Model file for the job. Use its own axes, mm. Face numbers are marked on the shaded views. A direction names the side the tool comes from. Round coordinates to 2 decimals unless told otherwise and drop trailing zeros. Order: outer loops, then holes, each group sorted by start corner. A loop starts at its lowest first (then second) coordinate and runs counter-clockwise, first axis right, second up. Notation, with made-up numbers: (-15, -15.5) - (26, -15.5) arc R20 cw to (26, 13.5) - close; hole circle Ø10 at (19, -28.5). An arc over 180 degrees is marked (long way). Write item = value, one per line.
```python
from build123d import *

# Parameters (mm, degrees)
SKETCH2_R                      = 70
BOSS_EXTRUDE1_DEPTH            = 15
CBORE_FOR_M5_SHCS1_D           = 5.5
CBORE_FOR_M5_SHCS1_CBORE_D     = 10
CBORE_FOR_M5_SHCS1_CBORE_DEPTH = 5
SKETCH23_R                     = 20.1
SKETCH23_R_2                   = 18.5
BOSS_EXTRUDE2_DEPTH            = 19
SKETCH24_R                     = 18.5
CUT_EXTRUDE4_DEPTH             = 101.801785698
SKETCH25_R                     = 22.2
SKETCH25_R_2                   = 20.1
BOSS_EXTRUDE3_DEPTH            = 4
FILLET2_R                      = 2


with BuildPart() as part:
    # Sketch2 → Boss-Extrude1 (new body)
    with BuildSketch(Plane(origin=(0, 0, 0), x_dir=(1, 0, 0), z_dir=(0, 1, 0))):
        with Locations(Location((0, 0, 0), (0, 0, 270))):
            Circle(SKETCH2_R)
    extrude(amount=BOSS_EXTRUDE1_DEPTH)

    # CBORE for M5 SHCS1 (through all)
    with Locations(Plane(origin=(0, 15, 0), x_dir=(1, 0, 0), z_dir=(0, 1, 0))):
        with Locations((0, 60), (60, 0), (-60, 0), (0, -60)):
            CounterBoreHole(CBORE_FOR_M5_SHCS1_D / 2, CBORE_FOR_M5_SHCS1_CBORE_D / 2, CBORE_FOR_M5_SHCS1_CBORE_DEPTH)

    # Sketch23 → Boss-Extrude2 (add)
    with BuildSketch(Plane(origin=(0, 15, 0), x_dir=(1, 0, 0), z_dir=(0, 1, 0))):
        with Locations(Location((0, 0, 0), (0, 0, 270))):
            Circle(SKETCH23_R)
        with Locations(Location((0, 0, 0), (0, 0, 270))):
            Circle(SKETCH23_R_2, mode=Mode.SUBTRACT)
    extrude(amount=BOSS_EXTRUDE2_DEPTH)

    # Sketch24 → Cut-Extrude4 (cut, through all)
    with BuildSketch(Plane(origin=(0, 15, 0), x_dir=(1, 0, 0), z_dir=(0, 1, 0))):
        with Locations(Location((0, 0, 0), (0, 0, 270))):
            Circle(SKETCH24_R)
    extrude(amount=-CUT_EXTRUDE4_DEPTH, mode=Mode.SUBTRACT)

    # Sketch25 → Boss-Extrude3 (add)
    with BuildSketch(Plane(origin=(0, 15, 0), x_dir=(1, 0, 0), z_dir=(0, 1, 0))):
        with Locations(Location((0, 0, 0), (0, 0, 270))):
            Circle(SKETCH25_R)
        with Locations(Location((0, 0, 0), (0, 0, 270))):
            Circle(SKETCH25_R_2, mode=Mode.SUBTRACT)
    extrude(amount=BOSS_EXTRUDE3_DEPTH)

    # Fillet2
    # the kernel refuses this fillet: 2 mm, written as the material it adds along each edge
    with BuildSketch(Plane(origin=(0, 15, 0), x_dir=(0, 0, 1), z_dir=(-1, 0, 0))) as fillet2_piece_1:
        with BuildLine():
            CenterArc((22.2 + FILLET2_R, FILLET2_R), FILLET2_R, 180, 90)
            Line((22.2, FILLET2_R), (22.2, 0))
            Line((22.2, 0), (22.2 + FILLET2_R, 0))
        make_face()
    revolve(axis=Axis((0, 15, 0), (0, 1, 0)))
    # the kernel refuses this fillet: 2 mm, written as the material it takes off along each edge
    with BuildSketch(Plane(origin=(0, 0, 0), x_dir=(0, 0, 1), z_dir=(-1, 0, 0))) as fillet2_2_piece_1:
        with BuildLine():
            CenterArc((70 - FILLET2_R, FILLET2_R), FILLET2_R, 270, 90)
            Line((70 - FILLET2_R, 0), (70, 0))
            Line((70, 0), (70, FILLET2_R))
        make_face()
    revolve(axis=Axis((0, 0, 0), (0, 1, 0)), mode=Mode.SUBTRACT)
    with BuildSketch(Plane(origin=(0, 34, 0), x_dir=(0, 0, 1), z_dir=(-1, 0, 0))) as fillet2_2_piece_2:
        with BuildLine():
            CenterArc((18.1, -1.959591794), FILLET2_R, 0, 78.463040967)
            Line((20.1, -1.959591794), (20.1, 0))
            Line((20.1, 0), (18.5, 0))
        make_face()
    revolve(axis=Axis((0, 34, 0), (0, 1, 0)), mode=Mode.SUBTRACT)
    with BuildSketch(Plane(origin=(0, 15, 0), x_dir=(0, 0, 1), z_dir=(-1, 0, 0))) as fillet2_2_piece_3:
        with BuildLine():
            CenterArc((70 - FILLET2_R, -FILLET2_R), FILLET2_R, 0, 90)
            Line((70 - FILLET2_R, 0), (70, 0))
            Line((70, 0), (70, -FILLET2_R))
        make_face()
    revolve(axis=Axis((0, 15, 0), (0, 1, 0)), mode=Mode.SUBTRACT)


solid = part.part
```
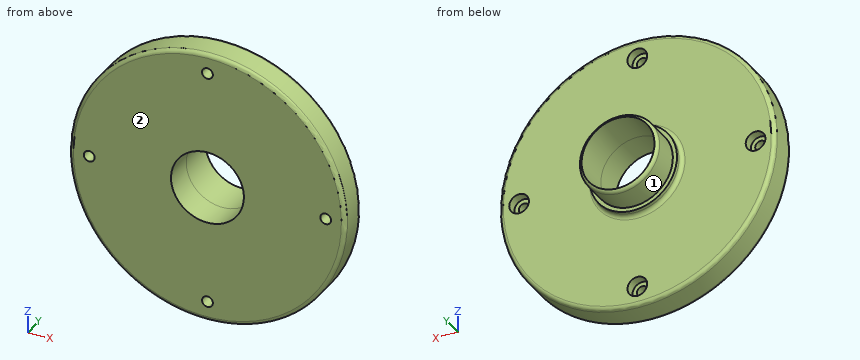
1) Cut at B-B (x = 0). Give the number of separate pieces and of enclosed holes in the cut face, and give its area (3 significant figures).
Conclusion:
separate_pieces = 4
enclosed_holes = 0
area = 1,410 mm^2
2) 3-axis set-ups, long thin cutter, end or side, ignore diameter. For the marked faces 1 and 2: which of +Z, -Z, +X, -X, +Y, -Y reach the whole face in a straight line?
Conclusion:
face_1 = +Y
face_2 = +Z, -Z, +X, -X, -Y
3) Wall check: line 1 along Y through (x, z) = (56, -30.5); line 2 along Z through (x, y) = (61.5, 6.5); line 3 along Z through (x, y) = (-11.5, 7.5). Give the ranges that are in metal, low to high.
Conclusion:
line_1 = 0 to 15
line_2 = -33.43 to -2.3, 2.3 to 33.43
line_3 = -69.05 to -14.49, 14.49 to 69.05
4) Flat gauge pins, fed straight in: pin 1 Ø11.5 at (x, z) = (0, 60) entering from -Y; pin 2 Ø5 at (x, y) = (-8, 21) entering from -Z; pin 3 Ø10 at (x, y) = (-41.5, 8) entering from -Z; pin 4 Ø3 at (x, y) = (44, 5.5) entering from -Z. Where does each tip first touch, or does it go through?
Conclusion:
pin_1 = 0
pin_2 = -21.23
pin_3 = -59.73
pin_4 = -55.62
5) Cut at A-A (y = 4). Write the cut outline in (x, z).
Conclusion:
outline = circle Ø140 at (0, 0); hole circle Ø5.5 at (-60, 0); hole circle Ø37 at (0, 0); hole circle Ø5.5 at (0, -60); hole circle Ø5.5 at (0, 60); hole circle Ø5.5 at (60, 0)
